```python
from build123d import *

# Parameters (mm, degrees)
BOSS_EXTRUDE1_DEPTH   = 15
M2_TAPPED_HOLE1_D     = 1.6
M2_TAPPED_HOLE1_DEPTH = 49.999
MIRROR2_COPY_1_D      = 1.6
MIRROR2_COPY_1_DEPTH  = 49.999


with BuildPart() as part:
    # Sketch1 → Boss-Extrude1 (new body)
    with BuildSketch(Plane.XY):
        Polygon((0, 0), (0, 54), (52, 54), (52, 0), (50, 0), (50, 52), (2, 52), (2, 0), align=None)
    extrude(amount=BOSS_EXTRUDE1_DEPTH)

    # M2 Tapped Hole1
    with Locations(Plane(origin=(52, 0, 0), x_dir=(0, 0, -1), z_dir=(1, 0, 0))):
        with Locations((-12, 2)):
            m2_tapped_hole1 = Hole(M2_TAPPED_HOLE1_D / 2, depth=M2_TAPPED_HOLE1_DEPTH)

    # Mirror1: M2 Tapped Hole1 across plane
    add(m2_tapped_hole1.mirror(Plane.XY.offset(7.5)), mode=Mode.SUBTRACT)

    # Mirror2: M2 Tapped Hole1 across plane
    add(m2_tapped_hole1.mirror(Plane(origin=(26, 0, 0), x_dir=(0, 0, 1), z_dir=(1, 0, 0))), mode=Mode.SUBTRACT)

    # Mirror2 copy 1
    with Locations(Plane(origin=(0, 0, 15), x_dir=(0, 0, 1), z_dir=(-1, 0, 0))):
        with Locations((-12, 2)):
            Hole(MIRROR2_COPY_1_D / 2, depth=MIRROR2_COPY_1_DEPTH)


solid = part.part
```
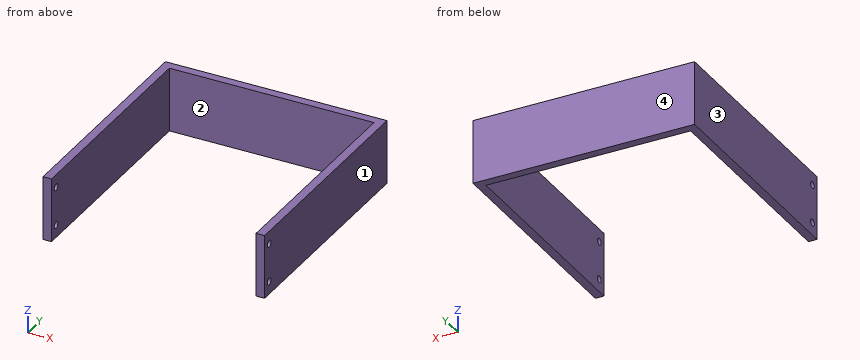
The model under review builds one solid part; all positions refer to its coordinate system, in mm. Face numbers are marked on the shaded views. Give positions to 0.01 mm unless a question says otherwise; leave off trailing zeros. Order: outer loops, then holes, each group sorted by start corner. A loop starts at its lowest first (then second) coordinate and runs counter-clockwise, first axis right, second up. Notation, with made-up numbers: (46.25, -27.75) - (71.25, -27.75) arc R14 cw to (71.25, -0.75) - close; hole circle Ø5 at (36, 47). An arc over 180 degrees is marked (long way). Use CSV: the item, a comma, the result in double quotes. Start each with the question number.
Q1. We need section B-B, the plane y = 2. Write out the cut boundary in (x, z).
Q2. We need section D-D, the plane x = 15.5. Write out the cut boundary in (y, z).
Q3. We need section C-C, the plane z = 12. Write out the cut boundary in (x, y), and give its area (3 significant figures).
Q4. To check wall thickness, follow line 1 along X through (y, z) = (24, 10.75); line 2 along Y through (x, z) = (0.75, 3); line 3 along Y through (x, z) = (6.5, 9). State the ranges of each line that lie inside material, in increasing order. Write a range as [from, to].
Q5. We need section A-A, the plane y = 13. Write out the cut boundary in (x, z).
Q6. Clearance check with a flat-ended pin moving along its axis: pin 1 Ø6 at (x, z) = (13, 13) entering from -Y. State where the tip first meets the part, or that it passes through.
Q7. The part is to be moulded in two halves that separate along X. For the marked faces 1, 2, 3 and 4, say which applies: +X half, -X half, draft (parallel to the pull), parting line (faces both ways), or undercut.
Outcome:
1,outline,"(0, 0) - (2, 0) - (2, 2.2) - (0, 2.2) - close; (0, 3.8) - (2, 3.8) - (2, 11.2) - (0, 11.2) - close; (0, 12.8) - (2, 12.8) - (2, 15) - (0, 15) - close; (50, 0) - (52, 0) - (52, 2.2) - (50, 2.2) - close; (50, 3.8) - (52, 3.8) - (52, 11.2) - (50, 11.2) - close; (50, 12.8) - (52, 12.8) - (52, 15) - (50, 15) - close"
2,outline,"(52, 0) - (54, 0) - (54, 15) - (52, 15) - close"
3,outline,"(0, 0) - (2, 0) - (2, 1.2) - (0, 1.2) - close; (0, 2.8) - (2, 2.8) - (2, 52) - (50, 52) - (50, 2.8) - (52, 2.8) - (52, 54) - (0, 54) - close; (50, 0) - (52, 0) - (52, 1.2) - (50, 1.2) - close"
3,area,"306 mm^2"
4,line 1,"x = [0, 2], [50, 52]"
4,line 2,"y = [0, 1.2], [2.8, 54]"
4,line 3,"y = [52, 54]"
5,outline,"(0, 0) - (2, 0) - (2, 15) - (0, 15) - close; (50, 0) - (52, 0) - (52, 15) - (50, 15) - close"
6,pin 1,"stops at y = 52"
7,face 1,"+X half"
7,face 2,"undercut"
7,face 3,"-X half"
7,face 4,"draft"
